Design review of the part built by this model. Coordinates are the model's own, in mm. A direction names the side the tool comes from. Give positions to 0.01 mm unless a question says otherwise; leave off trailing zeros. Order: outer loops, then holes, each group sorted by start corner. A loop starts at its lowest first (then second) coordinate and runs counter-clockwise, first axis right, second up.
```python
from build123d import *

# Parameters (mm, degrees)
SKETCH2_W           = 50
SKETCH2_H           = 50
SKETCH2_R           = 2
BOSS_EXTRUDE1_DEPTH = 2
SKETCH4_R           = 4.812837504
BOSS_EXTRUDE2_DEPTH = 2
BOSS_EXTRUDE3_START = 2
SKETCH3_R           = 4.812837504
BOSS_EXTRUDE3_DEPTH = 2
FILLET1_R           = 1
FILLET2_R           = 1


with BuildPart() as part:
    # Sketch2 → Boss-Extrude1 (new body)
    with BuildSketch(Plane(origin=(0, 0, 0), x_dir=(1, 0, 0), z_dir=(0, 1, 0))):
        Rectangle(SKETCH2_W, SKETCH2_H)
        with Locations(Location((0, 0, 0), (0, 0, 270))):
            Circle(SKETCH2_R, mode=Mode.SUBTRACT)
    extrude(amount=BOSS_EXTRUDE1_DEPTH)

    # Sketch4 → Boss-Extrude2 (add)
    with BuildSketch(Plane.ZY.offset(25)):
        Polygon((25, 2), (-25, 2), (-25, 0.026324244), (20, -58), (70, -58), align=None)
        with Locations(Location((40, -48, 0), (0, 0, 180))):
            Circle(SKETCH4_R, mode=Mode.SUBTRACT)
    extrude(amount=BOSS_EXTRUDE2_DEPTH)

    # Sketch3 → Boss-Extrude3 (add)
    with BuildSketch(Plane(origin=(25, 0, 0), x_dir=(0, 0, -1), z_dir=(1, 0, 0)).offset(BOSS_EXTRUDE3_START)):
        Polygon((-25, 2), (-70, -58), (-20, -58), (25, 0), (25, 2), align=None)
        with Locations((-40, -48)):
            Circle(SKETCH3_R, mode=Mode.SUBTRACT)
    extrude(amount=-BOSS_EXTRUDE3_DEPTH)

    # Fillet1
    fillet1_edges = [part.edges().sort_by_distance(p)[0] for p in [
        (-26, -58, 20),
        (26, -58, 20),
    ]]
    fillet(fillet1_edges, radius=FILLET1_R)

    # Fillet2
    fillet2_edges = [part.edges().sort_by_distance(p)[0] for p in [
        (-26, -58, 70),
        (26, -58, 70),
    ]]
    fillet(fillet2_edges, radius=FILLET2_R)


solid = part.part
```
1. Draft analysis for pull direction X (two halves, no side actions). For faces 4 (the face through (-2, 1, 0)), 5 (the face through (26, -26.8, 46.6)), 6 (the face through (27, -28, 23)), state which applies: pulls with the +X half, pulls with the -X half, needs draft (parallel to the pull), parting line crosses it, or undercut.
Recorded:
face 4: undercut
face 5: needs draft
face 6: pulls with the +X half
2. Take a section at A-A (x = 0). State the section outline as (y, z) points, then the cut area to 3 significant figures.
Recorded:
outline: (0, -25) - (2, -25) - (2, -2) - (0, -2) - close; (0, 2) - (2, 2) - (2, 25) - (0, 25) - close
area: 92.0 mm2
3. Machinability: for faces 1 (the face through (-27, -28, 21)), 2 (the face through (0, 1, 25)), 3 (the face through (0, 0, -6)), which of the approach directions +Z, -Z, +X, -X, +Y, -Y give a long, thin tool a straight path to every point of the face, cutting with its end or side? Answer none if there is none.
Recorded:
face 1: +Z, -Z, -X, +Y, -Y
face 2: +Z, +Y, -Y
face 3: +Z, -Z, -Y
4. For line 1 along X through (y, z) = (1.15, 0); line 2 along X through (y, z) = (-17, 33.5); line 3 along Y through (x, z) = (-8, 21), list the stretches that pass through material, from the lowest coordinate up.
Recorded:
line 1: x = -27 to -2, 2 to 27
line 2: x = -27 to -25, 25 to 27
line 3: y = 0 to 2
5. Take a section at B-B (z = 40). State the section outline as (x, y) points.
Recorded:
outline: (-27, -58) - (-25, -58) - (-25, -52.81) - (-27, -52.81) - close; (-27, -43.19) - (-25, -43.19) - (-25, -18) - (-27, -18) - close; (25, -58) - (27, -58) - (27, -52.81) - (25, -52.81) - close; (25, -43.19) - (27, -43.19) - (27, -18) - (25, -18) - close
6. For pin 1 (2 mm diameter, centred on x = -8, y = 1, fed in from +Z); pin 2 (6.5 mm diameter, centred on x = 0, z = 0, fed in from -Y), all flat-tipped, find the tip position at first contact; note any pin that passes through.
Recorded:
pin 1: stops at z = 25
pin 2: stops at y = 0
7. Take a section at D-D (z = 0). State the section outline as (x, y) points, then the cut area to 3 significant figures.
Recorded:
outline: (-27, -32.21) - (-25, -32.21) - (-25, 0) - (-2, 0) - (-2, 2) - (-27, 2) - close; (2, 0) - (25, 0) - (25, -32.22) - (27, -32.22) - (27, 2) - (2, 2) - close
area: 229 mm2
8. Take a section at C-C (y = -40.5). State the section outline as (x, z) points (3 decimals), then the cut area to 3 significant figures.
Recorded:
outline: (-27, 6.429) - (-25, 6.429) - (-25, 56.875) - (-27, 56.875) - close; (25, 6.422) - (27, 6.422) - (27, 56.875) - (25, 56.875) - close
area: 202 mm2
